from build123d import *

# Parameters (mm, degrees)
SKETCH1_R           = 2.5
BOSS_EXTRUDE1_DEPTH = 100
CUT_EXTRUDE1_START  = -0.64
SKETCH2_R           = 2.5
SKETCH2_R_2         = 2
CUT_EXTRUDE1_DEPTH  = 0.64
CUT_EXTRUDE2_START  = -0.64
SKETCH3_R           = 2.5
SKETCH3_R_2         = 2
CUT_EXTRUDE2_DEPTH  = 0.64
CUT_EXTRUDE3_START  = 51.86
SKETCH4_R           = 2.5
CUT_EXTRUDE3_DEPTH  = 51.86
CUT_EXTRUDE4_START  = 0.64
SKETCH6_R           = 2.5
SKETCH6_R_2         = 2
CUT_EXTRUDE4_DEPTH  = 0.64


with BuildPart() as part:
    # Sketch1 → Boss-Extrude1 (new body)
    with BuildSketch(Plane(origin=(0, 0, 0), x_dir=(0, 0, -1), z_dir=(1, 0, 0))):
        Circle(SKETCH1_R)
    extrude(amount=BOSS_EXTRUDE1_DEPTH)

    # Sketch2 → Cut-Extrude1 (cut)
    with BuildSketch(Plane(origin=(92, 0, 0), x_dir=(0, 0, -1), z_dir=(1, 0, 0)).offset(CUT_EXTRUDE1_START)):
        Circle(SKETCH2_R)
        Circle(SKETCH2_R_2, mode=Mode.SUBTRACT)
    extrude(amount=CUT_EXTRUDE1_DEPTH, mode=Mode.SUBTRACT)

    # Sketch3 → Cut-Extrude2 (cut)
    with BuildSketch(Plane(origin=(69.36, 0, 0), x_dir=(0, 0, -1), z_dir=(1, 0, 0)).offset(CUT_EXTRUDE2_START)):
        Circle(SKETCH3_R)
        Circle(SKETCH3_R_2, mode=Mode.SUBTRACT)
    extrude(amount=CUT_EXTRUDE2_DEPTH, mode=Mode.SUBTRACT)

    # Sketch4 → Cut-Extrude3 (cut)
    with BuildSketch(Plane.ZY.offset(-51.86).offset(CUT_EXTRUDE3_START)):
        Circle(SKETCH4_R)
    extrude(amount=-CUT_EXTRUDE3_DEPTH, mode=Mode.SUBTRACT)

    # Sketch6 → Cut-Extrude4 (cut)
    with BuildSketch(Plane.ZY.offset(-60.185).offset(CUT_EXTRUDE4_START)):
        Circle(SKETCH6_R)
        with Locations(Location((0, 0, 0), (0, 0, 180))):
            Circle(SKETCH6_R_2, mode=Mode.SUBTRACT)
    extrude(amount=-CUT_EXTRUDE4_DEPTH, mode=Mode.SUBTRACT)


solid = part.part
Here's how the part is built. I have some questions about the finished solid (model axes, mm). A direction names the side the tool comes from. Coordinates: 2 decimals unless noted, no trailing zeros. Write each loop counter-clockwise with the first axis right and the second up, starting at its lowest first coordinate (ties: lowest second). Pieces come first, ordered by that corner, then holes.
Item 1: On a 3-axis mill with a long thin cutter (end or side, diameter ignored), from which of +Z, -Z, +X, -X, +Y, -Y can I reach the whole of each face in a straight line? I mean faces 5 (the flat face through (51.86, 0, 0)), 6 (the cylindrical face through (91.676, -1.952, 0.434)). Say none if no direction works.
Item 2: If I drill on line 1 (X direction, y = -0.3, z = 2.25) (3 decimals); line 2 (Y direction, x = 68, z = -0.1), over which ranges is the centre line in solid material (lowest first)?
Item 3: I want a section at A-A on z = 0.4. Write out the boundary of the cut face in (x, y) (3 decimals), and give its area (3 significant figures).
Item 4: I want a section at B-B on x = 89. Write out the boundary of the cut face in (y, z), and give its area (3 significant figures).
Item 5: If we mould it in two halves opening along X, with no side actions, what happens to faces 1 (the flat face through (69.36, 2, 1)), 2 (the flat face through (100, 0, 0)), 3 (the flat face through (92, 2, 1)), 4 (the cylindrical face through (64.39, -2.44, 0.54))? For each: +X half, -X half, draft (parallel to the pull), parting line (faces both ways), or undercut.
Item 6: Will this pin go through, and if not, where does the flat tip stop? pin 1 (1.5 mm diameter, centred on x = 68, z = -1.5, fed in from +Y).
Findings below:
1. face 5: +Z, -Z, -X, +Y, -Y
1. face 6: none
2. line 1: x = 51.86 to 59.545, 60.185 to 68.72, 69.36 to 91.36, 92 to 100
2. line 2: y = -2.5 to 2.5
3. outline: (51.86, -2.468) - (59.545, -2.468) - (59.545, -1.96) - (60.185, -1.96) - (60.185, -2.468) - (68.72, -2.468) - (68.72, -1.96) - (69.36, -1.96) - (69.36, -2.468) - (91.36, -2.468) - (91.36, -1.96) - (92, -1.96) - (92, -2.468) - (100, -2.468) - (100, 2.468) - (92, 2.468) - (92, 1.96) - (91.36, 1.96) - (91.36, 2.468) - (69.36, 2.468) - (69.36, 1.96) - (68.72, 1.96) - (68.72, 2.468) - (60.185, 2.468) - (60.185, 1.96) - (59.545, 1.96) - (59.545, 2.468) - (51.86, 2.468) - close
3. area: 236 mm2
4. outline: circle Ø5 at (0, 0)
4. area: 19.6 mm2
5. face 1: undercut
5. face 2: +X half
5. face 3: undercut
5. face 4: draft
6. pin 1: stops at y = 2.38
